Here's how the part is built. I have some questions about the finished solid (model axes, mm). Face numbers are marked on the shaded views. A direction names the side the tool comes from. Coordinates: 2 decimals unless noted, no trailing zeros. Write each loop counter-clockwise with the first axis right and the second up, starting at its lowest first coordinate (ties: lowest second). Pieces come first, ordered by that corner, then holes.
Item 1: If we section it at B-B (y = 5): Please give me the cut outline in (x, z) (3 decimals).
Item 2: For the marked faces 1, 2 and 3, which set-ups out of +Z, -Z, +X, -X, +Y, -Y let a thin tool reach every point of the face, with its end or its side?
Item 3: If we section it at C-C (z = 18): Please give me the cut outline in (x, y), then the cut area to 3 significant figures.
Item 4: If we section it at A-A (z = 30): Please give me the cut outline in (x, y) (3 decimals).
Item 5: If I drill on line 1 (Y direction, x = 2, z = 30); line 2 (Z direction, x = 9.7, y = 15) (3 decimals); line 3 (Z direction, x = 5.75, y = 15), over which ranges is the centre line in solid material (lowest first)?
Item 6: I'm going to push flat-ended pins straight in: pin 1 Ø2 at (y, z) = (15.5, 10.5) entering from +X; pin 2 Ø5.5 at (y, z) = (15, 10) entering from +X; pin 3 Ø7.5 at (y, z) = (16.5, 29.5) entering from +X; pin 4 Ø3 at (x, y) = (46, -3.5) entering from -Z. Where does each tip first touch, or does it pass through?
Item 7: If we section it at D-D (y = 15): Please give me the cut outline in (x, z) (3 decimals).
Autodesk Inventor part; units mm, degrees
ref_plane "YZ Plane" through (0, 0, 0) normal (1, 0, 0) x (0, 1, 0)
ref_plane "XZ Plane" through (0, 0, 0) normal (0, 1, 0) x (-1, 0, 0)
ref_plane "XY Plane" through (0, 0, 0) normal (0, 0, 1) x (1, 0, 0)
sketch "Sketch1" plane through (0, 0, 0) normal (0, 0, 1) x (1, 0, 0)
  line L0 (0, 0) -> (10, 0)
  line L1 (10, 0) -> (10, 20)
  line L2 (10, 20) -> (0, 20)
  line L3 (0, 20) -> (0, 0)
  line L4 (10, 0) -> (-15, 0)
  line L5 (-15, 0) -> (-15, -10)
  line L6 (-15, -10) -> (10, -10)
  line L7 (10, -10) -> (10, 0)
  line L8 (10, -10) -> (60, -10)
  line L9 (60, -10) -> (60, 0)
  line L10 (60, 0) -> (10, 0)
  line L11 (10, 0) -> (10, -10)
  dimension "d0" = 10
  dimension "d1" = 20
  dimension "d2" = 25
  dimension "d3" = 10
  dimension "d4" = 50
extrude "Extrusion1" add sketch "Sketch1" along normal blind 40
sketch "Sketch2" plane through (10, 20, 40) normal (1, 0, 0) x (0, 0, -1)
  line L0 (40, 0) -> (0, 0) construction
  line L1 (40, -20) -> (0, -20) construction
  line L2 (0, -20) -> (0, 0) construction
  line L3 (0, 0) -> (40, 0) construction
  line L4 (40, 0) -> (40, -20) construction
  line L5 (40, 0) -> (40, -20) construction
  line L6 (0, 0) -> (40, -20) construction
  line L7 (0, 0) -> (0, -20) construction
  line L8 (40, 0) -> (0, -20) construction
  line L9 (10, -15) -> (30, -15) construction
  line L10 (30, -15) -> (30, -5) construction
  line L11 (30, -5) -> (10, -5) construction
  line L12 (10, -5) -> (10, -15) construction
  line L13 (10, -15) -> (30, -5) construction
  line L14 (30, -15) -> (10, -5) construction
  point P0 (20, -10)
  dimension "d9" = 20
hole "Hole1" at (10, 15, 30) at (10, 15, 10) at (10, 5, 10) at (10, 5, 30) direction (-1, 0, 0) diameter 3.9 end through all counterbore diameter 6.75 counterbore depth 1
fillet "Fillet3" radius 7.25 1 edges at (10, 0, 20)
properties part number "Test Stand"
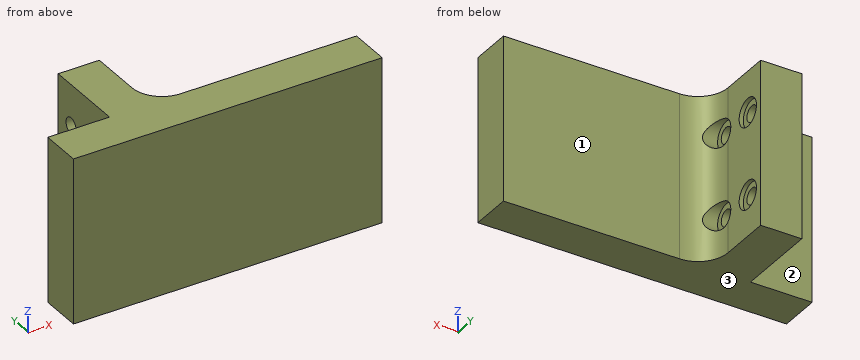
Answer list:
1. outline: (0, 0) - (10.358, 0) - (10.358, 6.625) - (9, 6.625) - (9, 8.05) - (0, 8.05) - close; (0, 11.95) - (9, 11.95) - (9, 13.375) - (10.358, 13.375) - (10.358, 26.625) - (9, 26.625) - (9, 28.05) - (0, 28.05) - close; (0, 31.95) - (9, 31.95) - (9, 33.375) - (10.358, 33.375) - (10.358, 40) - (0, 40) - close
2. face 1: +Z, -Z, +X, +Y
2. face 2: +Z, -Z, -X, +Y
2. face 3: -Z, +X, -X, +Y, -Y
3. outline: (-15, -10) - (60, -10) - (60, 0) - (17.25, 0) arc R7.25 cw to (10, 7.25) - (10, 20) - (0, 20) - (0, 0) - (-15, 0) - close
3. area: 961 mm2
4. outline: (-15, -10) - (60, -10) - (60, 0) - (17.25, 0) arc R7.25 cw to (12.676, 1.625) - (9, 1.625) - (9, 3.05) - (0, 3.05) - (0, 0) - (-15, 0) - close; (0, 6.95) - (9, 6.95) - (9, 8.375) - (10, 8.375) - (10, 11.625) - (9, 11.625) - (9, 13.05) - (0, 13.05) - close; (0, 16.95) - (9, 16.95) - (9, 18.375) - (10, 18.375) - (10, 20) - (0, 20) - close
5. line 1: y = -10 to 3.05, 6.95 to 13.05, 16.95 to 20
5. line 2: z = 0 to 6.625, 13.375 to 26.625, 33.375 to 40
5. line 3: z = 0 to 8.05, 11.95 to 28.05, 31.95 to 40
6. pin 1: passes through
6. pin 2: stops at x = 9
6. pin 3: stops at x = 10
6. pin 4: stops at z = 0
7. outline: (0, 0) - (10, 0) - (10, 6.625) - (9, 6.625) - (9, 8.05) - (0, 8.05) - close; (0, 11.95) - (9, 11.95) - (9, 13.375) - (10, 13.375) - (10, 26.625) - (9, 26.625) - (9, 28.05) - (0, 28.05) - close; (0, 31.95) - (9, 31.95) - (9, 33.375) - (10, 33.375) - (10, 40) - (0, 40) - close
